Model file for the job. Use its own axes, mm. A direction names the side the tool comes from. Coordinates: 2 decimals unless noted, no trailing zeros. Write each loop counter-clockwise with the first axis right and the second up, starting at its lowest first coordinate (ties: lowest second). Pieces come first, ordered by that corner, then holes. Notation, with made-up numbers: M -31,62.25 L -11,62.25 A19 ccw -11,73.25 Z; hole C 48.25,64.25 d7. An arc over 180 degrees is marked long. One line per question, with ' | ' between items. Start each with the question number.
(1) Cut at C-C (z = -51). Write the cut outline in (x, y), plus the area to 3 significant figures.
(2) Flat gauge pins, fed straight in: pin 1 Ø3 at (y, z) = (2, -130) entering from -X; pin 2 Ø1.6 at (y, z) = (35.5, -70.5) entering from -X; pin 3 Ø3 at (x, y) = (129, 39) entering from -Z; pin 4 Ø8 at (y, z) = (11.5, -18) entering from -X. Where does each tip first touch, or does it go through?
(3) Two-plate mould, pull along X, no slides. Class faces 1 (the face through (0, 2, -55)), 2 (the face through (148.971, 2, -126)), 3 (the face through (2, 2, -110.617)): +X half, -X half, draft (parallel to the pull), parting line (faces both ways), or undercut.
(4) Wall check: probe 1 along Y at (x, z) = (108.5, -72.5); probe 2 along Y at (x, z) = (78, -96.5); probe 3 along Z at (x, y) = (16.5, 51.5). Give the ranges that are in metal, low to high.
(5) Cut at B-B (x = 71.5). Write the cut outline in (y, z) (3 decimals), plus the area to 3 significant figures.
(6) Tool access for faces 4 (the face through (3.429, 2, -126)), 5 (the face through (151, 2, -110.617)), 6 (the face through (76, 53, -66.548)), 7 (the face through (76, 53, -76.073)): list every direction of +Z, -Z, +X, -X, +Y, -Y with a clear straight run to the whole face (end or side of a thin tool).
(7) Cut at D-D (z = -131.5). Write the cut outline in (x, y).
(8) Cut at A-A (y = 28). Write the cut outline in (x, z) (3 decimals), plus the area to 3 significant figures.
from build123d import *

# Parameters (mm, degrees)
SKETCH1_W           = 152.4
SKETCH1_H           = 142.621
BOSS_EXTRUDE1_DEPTH = 3.81
SKETCH2_W           = 127
SKETCH2_H           = 9.525
BOSS_EXTRUDE2_DEPTH = 57.15
CUT_EXTRUDE1_REACH  = 182.912
SKETCH3_W           = 101.6
SKETCH3_H           = 44.45
FILLET1_R           = 3.175
SKETCH4_W           = 3.429
SKETCH4_H           = 32.004
CUT_EXTRUDE2_DEPTH  = 217.408484448


with BuildPart() as part:
    # Sketch1 → Boss-Extrude1 (new body)
    with BuildSketch(Plane(origin=(0, 0, 0), x_dir=(1, 0, 0), z_dir=(0, 1, 0))):
        with Locations((76.2, 71.3105)):
            Rectangle(SKETCH1_W, SKETCH1_H)
    extrude(amount=BOSS_EXTRUDE1_DEPTH)

    # Sketch2 → Boss-Extrude2 (add)
    with BuildSketch(Plane(origin=(0, 3.81, 0), x_dir=(1, 0, 0), z_dir=(0, 1, 0))):
        with Locations((76.2, 71.3105)):
            Rectangle(SKETCH2_W, SKETCH2_H)
    extrude(amount=BOSS_EXTRUDE2_DEPTH)

    # Sketch3 → Cut-Extrude1 (cut, up to next)
    with BuildSketch(Plane.XY.offset(-66.548), mode=Mode.PRIVATE) as cut_extrude1_sk1:
        with Locations((76.2, 26.035)):
            Rectangle(SKETCH3_W, SKETCH3_H)
    cut_extrude1_tool1 = extrude(cut_extrude1_sk1.sketch, amount=-CUT_EXTRUDE1_REACH, mode=Mode.PRIVATE) & part.part
    add(cut_extrude1_tool1.solids().sort_by_distance((76.2, 26.035, -66.548))[0], mode=Mode.SUBTRACT)

    # Fillet1
    fillet1_edges = [part.edges().sort_by_distance(p)[0] for p in [
        (12.7, 3.81, -71.3105),
        (12.7, 32.385, -76.073),
        (19.05, 3.81, -66.548),
        (12.7, 32.385, -66.548),
        (139.7, 3.81, -71.3105),
        (139.7, 32.385, -66.548),
        (133.35, 3.81, -76.073),
        (139.7, 32.385, -76.073),
        (12.7, 60.96, -71.3105),
        (76.2, 60.96, -66.548),
        (139.7, 60.96, -71.3105),
        (76.2, 60.96, -76.073),
        (19.05, 3.81, -76.073),
        (133.35, 3.81, -66.548),
        (25.4, 26.035, -76.073),
        (76.2, 48.26, -76.073),
        (127, 26.035, -76.073),
        (25.4, 3.81, -71.3105),
        (25.4, 48.26, -71.3105),
        (127, 48.26, -71.3105),
        (127, 3.81, -71.3105),
        (25.4, 26.035, -66.548),
        (127, 26.035, -66.548),
        (76.2, 48.26, -66.548),
    ]]
    fillet(fillet1_edges, radius=FILLET1_R)

    # Sketch4 → Cut-Extrude2 (cut, through all)
    with BuildSketch(Plane(origin=(0, 3.81, 0), x_dir=(1, 0, 0), z_dir=(0, 1, 0))):
        with Locations((1.7145, 126.619)):
            Rectangle(SKETCH4_W, SKETCH4_H)
        with Locations((150.6855, 126.619)):
            Rectangle(SKETCH4_W, SKETCH4_H)
    extrude(amount=-CUT_EXTRUDE2_DEPTH, mode=Mode.SUBTRACT)


solid = part.part
Filled in:
1) outline: M 0,0 L 152.4,0 L 152.4,3.81 L 0,3.81 Z | area: 581 mm²
2) pin 1: x = 3.43 | pin 2: x = 12.7 | pin 3: z = -76.07 | pin 4: through
3) face 1: -X half | face 2: +X half | face 3: draft
4) probe 1: 0 to 3.81, 48.26 to 60.96 | probe 2: 0 to 3.81 | probe 3: -76.07 to -66.55
5) outline: M 0,-142.621 L 3.81,-142.621 L 3.81,0 L 0,0 Z; M 48.26,-72.898 A3.175 ccw 51.435,-76.073 L 57.785,-76.073 A3.175 ccw 60.96,-72.898 L 60.96,-69.723 A3.175 ccw 57.785,-66.548 L 51.435,-66.548 A3.175 ccw 48.26,-69.723 Z | area: 656 mm²
6) face 4: -Z, -X, +Y, -Y | face 5: -Z, +X, +Y, -Y | face 6: +Z, +X, -X, +Y | face 7: -Z, +X, -X, +Y
7) outline: M 3.43,0 L 148.97,0 L 148.97,3.81 L 3.43,3.81 Z
8) outline: M 12.7,-72.898 A3.175 ccw 15.875,-76.073 L 22.225,-76.073 A3.175 ccw 25.4,-72.898 L 25.4,-69.723 A3.175 ccw 22.225,-66.548 L 15.875,-66.548 A3.175 ccw 12.7,-69.723 Z; M 127,-72.898 A3.175 ccw 130.175,-76.073 L 136.525,-76.073 A3.175 ccw 139.7,-72.898 L 139.7,-69.723 A3.175 ccw 136.525,-66.548 L 130.175,-66.548 A3.175 ccw 127,-69.723 Z | area: 225 mm²
